from build123d import *

# Parameters (mm, degrees)
SKETCH1_W           = 20
SKETCH1_H           = 10
BOSS_EXTRUDE1_DEPTH = 20
SKETCH3_R           = 3
CUT_EXTRUDE1_DEPTH  = 10
SKETCH4_R           = 1
CUT_EXTRUDE2_DEPTH  = 1
SKETCH7_R           = 3
CUT_EXTRUDE10_DEPTH = 20
SKETCH8_R           = 1.5
SKETCH8_R_2         = 0.75
CUT_EXTRUDE11_DEPTH = 4


with BuildPart() as part:
    # Sketch1 → Boss-Extrude1 (new body)
    with BuildSketch(Plane.XY):
        Rectangle(SKETCH1_W, SKETCH1_H)
    extrude(amount=BOSS_EXTRUDE1_DEPTH)

    # Sketch3 → Cut-Extrude1 (cut)
    with BuildSketch(Plane(origin=(0, 5, 0), x_dir=(1, 0, 0), z_dir=(0, 1, 0))):
        with Locations(Location((0, -5, 0), (0, 0, 270))):
            Circle(SKETCH3_R)
    extrude(amount=-CUT_EXTRUDE1_DEPTH, mode=Mode.SUBTRACT)

    # Sketch4 → Cut-Extrude2 (cut)
    with BuildSketch(Plane(origin=(0, 5, 0), x_dir=(1, 0, 0), z_dir=(0, 1, 0))):
        with Locations(Location((0, -15, 0), (0, 0, 270))):
            Circle(SKETCH4_R)
    extrude(amount=-CUT_EXTRUDE2_DEPTH, mode=Mode.SUBTRACT)

    # Sketch7 → Cut-Extrude10 (cut)
    with BuildSketch(Plane(origin=(10, 0, 0), x_dir=(0, 0, -1), z_dir=(1, 0, 0))):
        with Locations((-15, 0)):
            Circle(SKETCH7_R)
    extrude(amount=-CUT_EXTRUDE10_DEPTH, mode=Mode.SUBTRACT)

    # Sketch8 → Cut-Extrude11 (cut)
    with BuildSketch(Plane(origin=(10, 0, 0), x_dir=(0, 0, -1), z_dir=(1, 0, 0))):
        with Locations((-7, 0)):
            Circle(SKETCH8_R)
        with Locations((-4.501923946, 2.710056555)):
            Circle(SKETCH8_R_2)
    extrude(amount=-CUT_EXTRUDE11_DEPTH, mode=Mode.SUBTRACT)


solid = part.part
Source: CAD feature listing. Evaluate the final solid. Frame: model axes, mm. A direction names the side the tool comes from. Round coordinates to 2 decimals unless told otherwise and drop trailing zeros. Loops run counter-clockwise (first coordinate to the right, second up) from the corner with the lowest first, then second, coordinate; pieces in that order, holes last. Notation, with made-up numbers: M 34,-12.75 L 39,-12.75 A31 cw 39,16.25 Z; hole C 11.5,51.5 d8. An arc over 180 degrees is marked long. Return JSON: item names as keys, results as strings. Group by question number.
1. Mould query, pull axis Z, two halves, no side actions, for faces 4 (the face through (0, 5, 10)), 5 (the face through (0, 0, 20)), 6 (the face through (-0.383, 4.507, 15.924)). Classes: released by +Z, released by -Z, zero draft, split by the parting line, or undercut.
2. Section query B-B on x = 0. Output: boundary loops of the cut face in (y, z), and give its area (3 significant figures).
3. Material intervals for line 1 along Y through (x, z) = (8.25, 4.5); line 2 along Y through (x, z) = (-2.25, 15); line 3 along X through (y, z) = (4.35, 15), sorted ascending. Write a range as from..to.
4. Reachability of faces 1 (the face through (6, 3, 5)), 2 (the face through (0, 4, 15)), 3 (the face through (-10, 0, 10)) from +Z, -Z, +X, -X, +Y, -Y: full face, straight path, thin tool, end or side. Return the list, or none.
5. Section query A-A on y = 0. Output: boundary loops of the cut face in (x, z), and give its area (3 significant figures).
6. Section query C-C on z = 15. Output: boundary loops of the cut face in (x, y).
7. Pin query (flat end, axial travel): pin 1 (9.5 mm diameter, centred on x = 0, z = 5, fed in from -Y); pin 2 (1.6 mm diameter, centred on x = 0, z = 15, fed in from +Y); pin 3 (1.5 mm diameter, centred on y = -0.5, z = 7.5, fed in from +X); pin 4 (3 mm diameter, centred on y = 0, z = 15.5, fed in from -X). Return the tip coordinate at first contact, or that it passes through.
8. Section query D-D on x = -8. Output: boundary loops of the cut face in (y, z).
Checks:
{
 "1": {"face 4": "zero draft", "face 5": "released by +Z", "face 6": "undercut"},
 "2": {"outline": "M -5,0 L 5,0 L 5,2 L -5,2 Z; M -5,8 L 5,8 L 5,14 L 4,14 L 4,16 L 5,16 L 5,20 L -5,20 Z; hole C 0,15 d6", "area": "110 mm²"},
 "3": {"line 1": "y = -5..1.96, 3.46..5", "line 2": "y = -5..-3, 3..5", "line 3": "x = -10..-1, 1..10"},
 "4": {"face 1": "+X", "face 2": "+Y", "face 3": "+Z, -Z, -X, +Y, -Y"},
 "5": {"outline": "M -10,0 L 10,0 L 10,5.5 L 6,5.5 L 6,8.5 L 10,8.5 L 10,12 L -10,12 Z; M -10,18 L 10,18 L 10,20 L -10,20 Z; hole C 0,5 d6", "area": "240 mm²"},
 "6": {"outline": "M -10,-5 L 10,-5 L 10,-3 L -10,-3 Z; M -10,3 L 10,3 L 10,5 L 1,5 L 1,4 L -1,4 L -1,5 L -10,5 Z"},
 "7": {"pin 1": "stops at y = -5", "pin 2": "stops at y = 4", "pin 3": "stops at x = 6", "pin 4": "passes through"},
 "8": {"outline": "M -5,0 L 5,0 L 5,20 L -5,20 Z; hole C 0,15 d6"}
}
